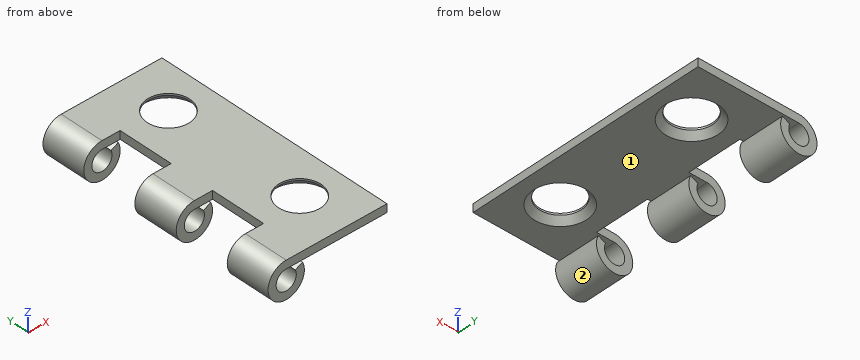
from build123d import *

# Parameters (mm, degrees)
EXTRUDE1_DEPTH          = 9.525
LPATTERN2_COUNT         = 2
LPATTERN2_PITCH         = 11.1125
CUT_EXTRUDE1_DEPTH      = 13.472746554
CUT_EXTRUDE1_DEPTH_BACK = 13.472746554
SKETCH4_W               = 2.8575
SKETCH4_H               = 4.318


with BuildPart() as part:
    # Sketch1 → Extrude1 (new, symmetric)
    with BuildSketch(Plane(origin=(0, 0, 0), x_dir=(1, 0, 0), z_dir=(0, 1, 0))):
        with BuildLine():
            Line((0, -0.79375), (7.9248, -0.79375))
            Line((7.9248, -0.79375), (7.9248, -1.42875))
            Line((7.9248, -1.42875), (0, -1.42875))
            ThreePointArc((0, -1.42875), (-0.753017368, 1.214204022), (1.279883418, -0.635))
            Line((1.279883418, -0.635), (0.711046343, -0.352777778))
            ThreePointArc((0.711046343, -0.352777778), (-0.418342982, 0.67455779), (0, -0.79375))
        make_face()
    extrude(amount=EXTRUDE1_DEPTH, both=True)

    # Sketch7 → Cut-Revolve1 (revolve, cut)
    with BuildSketch(Plane(origin=(4.7498, 0, 0), x_dir=(0, 0, -1), z_dir=(1, 0, 0)), mode=Mode.PRIVATE) as cut_revolve1_sk:
        Polygon((-0.79375, 5.55625), (-0.79375, 7.65175), (-1.290479078, 7.21995), (-1.42875, 7.21995), (-1.42875, 5.55625), align=None)
    cut_revolve1 = revolve(cut_revolve1_sk.sketch.rotate(Axis((4.7498, 5.55625, -1.822321443), (0, 0, 1)), 90), axis=Axis((4.7498, 5.55625, -1.822321443), (0, 0, 1)), mode=Mode.SUBTRACT)

    # LPattern2: Cut-Revolve1 ×2
    with Locations(*[(0, -i * LPATTERN2_PITCH, 0) for i in range(1, LPATTERN2_COUNT)]):
        add(cut_revolve1, mode=Mode.SUBTRACT)

    # Sketch4 → Cut-Extrude1 (cut, two sides: drawn at the far end of the back side and taken through both)
    with BuildSketch(Plane.XY.offset(-CUT_EXTRUDE1_DEPTH_BACK)):
        with Locations((0, 3.9116)):
            Rectangle(SKETCH4_W, SKETCH4_H)
        with Locations((0, -3.9116)):
            Rectangle(SKETCH4_W, SKETCH4_H)
    extrude(amount=CUT_EXTRUDE1_DEPTH + CUT_EXTRUDE1_DEPTH_BACK, mode=Mode.SUBTRACT)


solid = part.part
Design review of the part built by this model. Coordinates are the model's own, in mm. Face numbers are marked on the shaded views. A direction names the side the tool comes from. Give positions to 0.01 mm unless a question says otherwise; leave off trailing zeros. Write each loop counter-clockwise with the first axis right and the second up, starting at its lowest first coordinate (ties: lowest second). Pieces come first, ordered by that corner, then holes. Notation, with made-up numbers: M -10,-26 L 13,-26 A22 ccw 13,13 Z; hole C -5,48.25 d2. An arc over 180 degrees is marked long. Answer as a JSON object with one key per item and string values. Group by question number.
1) For line 1 along Y through (x, z) = (1, -0.65) (3 decimals); line 2 along Y through (x, z) = (5, 1.35) (3 decimals); line 3 along Z through (x, y) = (0, -8.45), list the stretches that pass through material, from the lowest coordinate up.
2) We need section C-C (y = -1). Give the boundary of the cut face in (x, z) (1 decimal), and give its area (3 significant figures).
3) Tool access review of the marked faces 1 and 2: name each direction out of +Z, -Z, +X, -X, +Y, -Y from which nothing blocks a thin tool from reaching the whole face with its end or side.
4) We need section B-B (z = -1). Give the boundary of the cut face in (x, y) (3 decimals).
5) Clearance check with flat-ended pins moving along their axes: pin 1 Ø0.7 at (y, z) = (-3, 1) entering from -X; pin 2 Ø4.5 at (x, y) = (4.75, -5.56) entering from -Z; pin 3 Ø5.5 at (x, y) = (4.75, 5.56) entering from +Z; pin 4 Ø1.5 at (y, z) = (6, 1) entering from -X. State where each tip first meets the part, or that it passes through.
6) We need section A-A (z = 0). Give the boundary of the cut face in (x, y) (3 decimals), and give its area (3 significant figures).
7) We need section D-D (y = -3.25). Give the boundary of the cut face in (x, z).
Answer key:
{
 "1": {"line 1": "y = -9.525 to -6.071, -1.753 to 1.753, 6.071 to 9.525", "line 2": "y = -9.525 to -7.201, -3.911 to 3.911, 7.201 to 9.525", "line 3": "z = -1.43 to -0.79, 0.79 to 1.43"},
 "2": {"outline": "M 0,0.8 L 7.9,0.8 L 7.9,1.4 L 0,1.4 A1.4 ccw long 1.3,0.6 L 0.7,0.4 A0.8 cw long Z", "area": "8.68 mm²"},
 "3": {"face 1": "+X, +Y, -Y", "face 2": "+Y, -Y"},
 "4": {"outline": "M -1.02,-9.525 L 1.02,-9.525 L 1.02,-6.071 L -1.02,-6.071 Z; M -1.02,-1.753 L 1.02,-1.753 L 1.02,1.753 L -1.02,1.753 Z; M -1.02,6.071 L 1.02,6.071 L 1.02,9.525 L -1.02,9.525 Z"},
 "5": {"pin 1": "stops at x = 1.43", "pin 2": "stops at z = 0.79", "pin 3": "stops at z = 1.43", "pin 4": "stops at x = -1.41"},
 "6": {"outline": "M -1.429,-9.525 L -0.794,-9.525 L -0.794,-6.071 L -1.429,-6.071 Z; M -1.429,-1.753 L -0.794,-1.753 L -0.794,1.753 L -1.429,1.753 Z; M -1.429,6.071 L -0.794,6.071 L -0.794,9.525 L -1.429,9.525 Z; M 0.794,-9.525 L 1.429,-9.525 L 1.429,-6.071 L 0.794,-6.071 Z; M 0.794,-1.753 L 1.429,-1.753 L 1.429,1.753 L 0.794,1.753 Z; M 0.794,6.071 L 1.429,6.071 L 1.429,9.525 L 0.794,9.525 Z", "area": "13.2 mm²"},
 "7": {"outline": "M 1.43,0.79 L 7.92,0.79 L 7.92,1.43 L 1.43,1.43 Z"}
}
